```python
from build123d import *

# Parameters (mm, degrees)
IZIM3_R                 = 1.25
KES_EKSTR_ZYON1_DEPTH   = 10
DAIRESEL_KAPLAMA2_COUNT = 4


with BuildPart() as part:
    # Çizim2 → Döndür1 (revolve)
    with BuildSketch(Plane.XY, mode=Mode.PRIVATE) as d_nd_r1_sk:
        Polygon((-14.222748097, 7), (98.777251903, 7), (98.777251903, 11), (105.777251903, 11), (105.777251903, 12), (85.777251903, 12), (85.777251903, 15), (80.777251903, 15), (70.777251903, 10), (0.777251903, 10), (-9.222748097, 22.5), (-14.222748097, 22.5), align=None)
    revolve(d_nd_r1_sk.sketch.rotate(Axis((0, 0, 0), (1, 0, 0)), 90), axis=Axis((0, 0, 0), (1, 0, 0)))

    # Çizim3 → Kes-Ekstrüzyon1 (cut)
    with BuildSketch(Plane.ZY.offset(14.222748097)):
        with Locations((0, 18.75)):
            Circle(IZIM3_R)
    kes_ekstr_zyon1 = extrude(amount=-KES_EKSTR_ZYON1_DEPTH, mode=Mode.SUBTRACT)

    # Dairesel Kaplama2: Kes-Ekstrüzyon1 ×4 about axis
    dairesel_kaplama2_axis = Axis((0, 0, 0), (1, 0, 0))
    for i in range(1, DAIRESEL_KAPLAMA2_COUNT):
        add(kes_ekstr_zyon1.rotate(dairesel_kaplama2_axis, i * 360 / DAIRESEL_KAPLAMA2_COUNT), mode=Mode.SUBTRACT)


solid = part.part
```
Input: part model. Units: mm. Frame: model coordinates. A direction names the side the tool comes from. Give positions to 0.01 mm unless a question says otherwise; leave off trailing zeros. Order: outer loops, then holes, each group sorted by start corner. A loop starts at its lowest first (then second) coordinate and runs counter-clockwise, first axis right, second up. Notation, with made-up numbers: M 33.5,18.25 L 57.5,18.25 A26 cw 57.5,43.25 Z; hole C -38,-9.75 d2. An arc over 180 degrees is marked long. Return JSON: item names as keys, results as strings.
1) Contact query for flat-ended pins moving along their axis: pin 1 (5 mm diameter, centred on x = 91.5, z = 4, fed in from -Y); pin 2 (8 mm diameter, centred on x = 11.5, y = 8, fed in from +Z); pin 3 (18 mm diameter, centred on y = 0, z = 0, fed in from +X). Output: stop coordinate, or through.
Taken from the geometry:
{"pin 1": "stops at y = -11.91", "pin 2": "stops at z = 9.17", "pin 3": "stops at x = 98.78"}
2) Access query for faces 4 (the face through (35, 0, -10)), 5 (the face through (-9.79, -0.27, -17.53)), 6 (the face through (95.637, -3.604, 11.446)). Directions: +Z, -Z, +X, -X, +Y, -Y. A direction counts if a zero-diameter tool reaches every point of the face in a straight line with its end or side. Return the directions, or none.
Taken from the geometry:
{"face 4": "none", "face 5": "+X, -X", "face 6": "+X"}
3) Section query A-A on y = 0. Count the separate pieces of the cut face and the enclosed holes in it, and give its area (3 significant figures).
Taken from the geometry:
{"separate pieces": "4", "enclosed holes": "0", "area": "1,050 mm2"}
4) Line query: L1, parallel to Y at x = 51, z = 0; L2, parallel to X at y = -7.5, z = -9; L3, parallel to Y at x = -10, z = -18. Output: solid intervals per line, ascending. Write a range as [from, to].
Taken from the geometry:
{"L1": "y = [-10, -7], [7, 10]", "L2": "x = [-14.22, -0.6], [74.21, 105.78]", "L3": "y = [-13.5, -1], [1, 13.5]"}
5) Section query C-C on x = 12. Output: boundary loops of the cut face in (y, z), and give its area (3 significant figures).
Taken from the geometry:
{"outline": "C 0,0 d20; hole C 0,0 d14", "area": "160 mm2"}
6) Section query D-D on x = 97.5. Output: boundary loops of the cut face in (y, z), and give its area (3 significant figures).
Taken from the geometry:
{"outline": "C 0,0 d24; hole C 0,0 d14", "area": "298 mm2"}
7) Mould query, pull axis Y, two halves, no side actions, for faces 1 (the face through (105.777, 10, -5)), 2 (the face through (-9.79, 17.53, -0.27)), 3 (the face through (83.24, -12.65, 8.06)). Classes: released by +Y, released by -Y, zero draft, split by the parting line, or undercut.
Taken from the geometry:
{"face 1": "zero draft", "face 2": "undercut", "face 3": "split by the parting line"}
